Could you check a few things on this model? Use its own coordinates, in mm. A direction names the side the tool comes from. Round coordinates to 2 decimals unless told otherwise and drop trailing zeros. Loops run counter-clockwise (first coordinate to the right, second up) from the corner with the lowest first, then second, coordinate; pieces in that order, holes last. Notation, with made-up numbers: (-24, -19) - (-7, -19) arc R16 cw to (-7, 5) - close; hole circle Ø10 at (13, -30.5). An arc over 180 degrees is marked (long way). Answer as CSV lines item,"result". Start each with the question number.
1) We'd pull the mould along Y, two halves only. Please class faces 1 (the face through (0, 149, 3)), 2 (the face through (-3, 146.05, 3)), 3 (the face through (61, 30.099, 3)): pulls with the +Y half, pulls with the -Y half, needs draft (parallel to the pull), parting line crosses it, or undercut.
2) Suppose I cut it at A-A, the plane y = 57.5. Write out the boundary of the cut face in (x, z), then the cut area to 3 significant figures.
3) Which directions (+Z, -Z, +X, -X, +Y, -Y) give clear straight access to the entire face, cutting with the end or side of a thin tool? Please do faces 4 (the face through (63.5, 149, 3)), 5 (the face through (54.61, 32, 3)), 6 (the face through (63.5, 3, 3)), 7 (the face through (8.89, 121, 3)).
4) I'm going to push flat-ended pins straight in: pin 1 Ø1.2 at (x, z) = (56.5, 3.5) entering from -Y; pin 2 Ø2 at (y, z) = (95.5, 5.5) entering from -X; pin 3 Ø2 at (y, z) = (52.5, 4) entering from +X; pin 4 Ø3 at (x, z) = (-2, 3) entering from -Y. Where does each tip first touch, or does it pass through?
5) Please list where these lines run through material, in increasing order: line 1 along Y through (x, z) = (-1.5, 4); line 2 along Y through (x, z) = (62, 2.25); line 3 along X through (y, z) = (65, 1.5).
```python
from build123d import *

# Parameters (mm, degrees)
SKETCH1_W           = 63.5
SKETCH1_H           = 152.4
BOSS_EXTRUDE1_DEPTH = 6.35
SKETCH2_W           = 6.35
SKETCH2_H           = 12.7
BOSS_EXTRUDE3_DEPTH = 6.35
SKETCH4_W           = 8.89
SKETCH4_H           = 3.302
SKETCH4_W_2         = 2.5
SKETCH4_H_2         = 6.5
CUT_EXTRUDE4_DEPTH  = 6.35


with BuildPart() as part:
    # Sketch1 → Boss-Extrude1 (new body)
    with BuildSketch(Plane.XY):
        with Locations((31.75, 76.2)):
            Rectangle(SKETCH1_W, SKETCH1_H)
    extrude(amount=BOSS_EXTRUDE1_DEPTH)

    # Sketch2 → Boss-Extrude3 (add)
    with BuildSketch(Plane.XY.offset(6.35)):
        with Locations((-3.175, 76.2)):
            Rectangle(SKETCH2_W, SKETCH2_H)
        with Locations((66.675, 139.7)):
            Rectangle(SKETCH2_W, SKETCH2_H)
        with Locations((66.675, 76.2)):
            Rectangle(SKETCH2_W, SKETCH2_H)
        with Locations((66.675, 12.7)):
            Rectangle(SKETCH2_W, SKETCH2_H)
        with Locations((-3.175, 12.7)):
            Rectangle(SKETCH2_W, SKETCH2_H)
        with Locations((-3.175, 139.7)):
            Rectangle(SKETCH2_W, SKETCH2_H)
    extrude(amount=-BOSS_EXTRUDE3_DEPTH)

    # Sketch4 → Cut-Extrude4 (cut)
    with BuildSketch(Plane.XY.offset(6.35)):
        with Locations((4.445, 120.65)):
            Rectangle(SKETCH4_W, SKETCH4_H)
        with Locations((6.37, 120.65)):
            Rectangle(SKETCH4_W_2, SKETCH4_H_2)
        with Locations((6.37, 31.75)):
            Rectangle(SKETCH4_W_2, SKETCH4_H_2)
        with Locations((4.445, 31.75)):
            Rectangle(SKETCH4_W, SKETCH4_H)
        with Locations((59.055, 31.75)):
            Rectangle(SKETCH4_W, SKETCH4_H)
        with Locations((57.13, 31.75)):
            Rectangle(SKETCH4_W_2, SKETCH4_H_2)
        with Locations((57.13, 120.65)):
            Rectangle(SKETCH4_W_2, SKETCH4_H_2)
        with Locations((59.055, 120.65)):
            Rectangle(SKETCH4_W, SKETCH4_H)
    extrude(amount=-CUT_EXTRUDE4_DEPTH, mode=Mode.SUBTRACT)


solid = part.part
```
Filled sheet:
1,face 1,"needs draft"
1,face 2,"pulls with the +Y half"
1,face 3,"undercut"
2,outline,"(0, 0) - (63.5, 0) - (63.5, 6.35) - (0, 6.35) - close"
2,area,"403 mm²"
3,face 4,"+Z, -Z, +X, +Y"
3,face 5,"+Z, -Z, +X"
3,face 6,"+Z, -Z, +X, -Y"
3,face 7,"+Z, -Z, -X"
4,pin 1,"y = 0"
4,pin 2,"x = 0"
4,pin 3,"x = 63.5"
4,pin 4,"y = 6.35"
5,line 1,"6.35 to 19.05, 69.85 to 82.55, 133.35 to 146.05"
5,line 2,"0 to 30.1, 33.4 to 119, 122.3 to 152.4"
5,line 3,"0 to 63.5"
